Geometry: final body of the model. Coordinates: model frame, mm. Face numbers are marked on the shaded views. Coordinates: 2 decimals unless noted, no trailing zeros. Order: outer loops, then holes, each group sorted by start corner. A loop starts at its lowest first (then second) coordinate and runs counter-clockwise, first axis right, second up. Notation, with made-up numbers: (-6.5, 56) - (23.5, 56) arc R20 ccw to (23.5, 68) - close; hole circle Ø2 at (83.5, 4.5). An arc over 180 degrees is marked (long way). Use a Markdown table: item, result. Add a question column.
```python
from build123d import *

# Parameters (mm, degrees)
SHELL1_T            = -3.81
SKETCH2_R           = 39.624
BOSS_EXTRUDE1_DEPTH = 88.9
SKETCH4_R           = 38.1
CUT_EXTRUDE1_DEPTH  = 88.9
SKETCH5_R           = 34.539650962
CUT_EXTRUDE2_DEPTH  = 575.240692351
SKETCH7_R           = 5.930093594
CUT_EXTRUDE5_DEPTH  = 571.44899759
SKETCH8_R           = 3.175
CUT_EXTRUDE6_DEPTH  = 486.842446429
CIRPATTERN1_COUNT   = 4


with BuildPart() as part:
    # Sketch1 → Revolve1 (revolve)
    with BuildSketch(Plane.XY, mode=Mode.PRIVATE) as revolve1_sk:
        Polygon((0, 0), (-39.624, 0), (0, 635), align=None)
    revolve(revolve1_sk.sketch.rotate(Axis((0, 635, 0), (0, -1, 0)), 180), axis=Axis((0, 635, 0), (0, -1, 0)))


with BuildPart() as body_2:
    # Split1: the piece on the far side of the plane
    add(part.part)
    split(bisect_by=Plane.ZX.offset(482.6), keep=Keep.BOTTOM)

    # Shell1
    shell1_openings = [body_2.faces().sort_by_distance(p)[0] for p in [
        (0, 0, 0),
    ]]
    offset(amount=SHELL1_T, openings=shell1_openings, kind=Kind.INTERSECTION)

    # Sketch2 → Boss-Extrude1 (add)
    with BuildSketch(Plane.XZ):
        Circle(SKETCH2_R)
    extrude(amount=BOSS_EXTRUDE1_DEPTH)

    # Sketch4 → Cut-Extrude1 (cut)
    with BuildSketch(Plane.XZ.offset(88.9)):
        Circle(SKETCH4_R)
    extrude(amount=-CUT_EXTRUDE1_DEPTH, mode=Mode.SUBTRACT)

    # Sketch7 → Cut-Extrude5 (cut, through all)
    with BuildSketch(Plane(origin=(0, 478.79, 0), x_dir=(-1, 0, 0), z_dir=(0, -1, 0))):
        with Locations(Location((0, 0, 0), (0, 0, 90))):
            Circle(SKETCH7_R)
    extrude(amount=-CUT_EXTRUDE5_DEPTH, mode=Mode.SUBTRACT)

    # Sketch8 → Cut-Extrude6 (cut, through all)
    with BuildSketch(Plane(origin=(0, 0, 0), x_dir=(0, 0, -1), z_dir=(1, 0, 0))):
        with Locations(Location((0, -47.625, 0), (0, 0, 270))):
            Circle(SKETCH8_R)
    cut_extrude6 = extrude(amount=CUT_EXTRUDE6_DEPTH, mode=Mode.SUBTRACT)

    # CirPattern1: Cut-Extrude6 ×4 about axis
    cirpattern1_axis = Axis((0, -88.9, 0), (0, 1, 0))
    for i in range(1, CIRPATTERN1_COUNT):
        add(cut_extrude6.rotate(cirpattern1_axis, i * 360 / CIRPATTERN1_COUNT), mode=Mode.SUBTRACT)


with BuildPart() as part_1:
    add(part.part)

    # Split1
    split(bisect_by=Plane.ZX.offset(482.6), keep=Keep.TOP)

    # Sketch5 → Cut-Extrude2 (cut, through all)
    with BuildSketch(Plane(origin=(0, 482.6, 0), x_dir=(1, 0, 0), z_dir=(0, 1, 0))):
        Circle(SKETCH5_R)
    extrude(amount=CUT_EXTRUDE2_DEPTH, mode=Mode.SUBTRACT)


solid = body_2.part
```
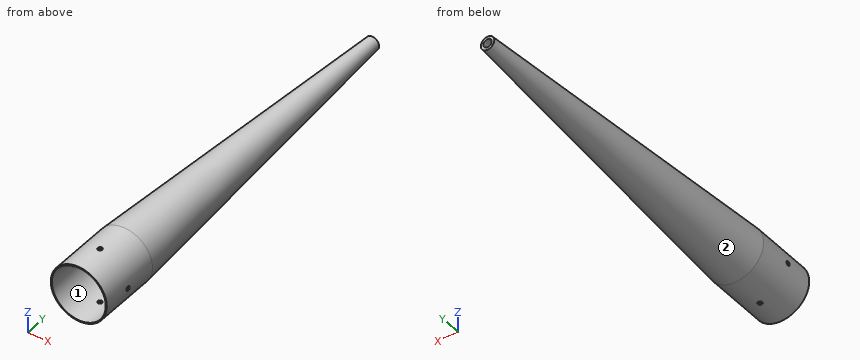
1) Line query: line 1 (Z direction, x = 0, y = -29); line 2 (Z direction, x = -26, y = -45.5); line 3 (X direction, y = 480.8, z = 0). Output: solid intervals per line, ascending. Write a range as from..to.
2) First-contact query: pin 1 (1.5 mm diameter, centred on x = -3.5, y = 153.5, fed in from +Z); pin 2 (6 mm diameter, centred on x = 2, y = 120, fed in from -Z); pin 3 (5 mm diameter, centred on y = 176.5, z = 13.5, fed in from +X). Flat tips, straight axial feed; report the tip coordinate or a pass-through.
3) Section query B-B (y = 287.5). Return the cut outline in (x, z), and give its area (3 significant figures).
4) Draft query along X for the marked faces 1 and 2. Return one class per face: released by +X, released by -X, zero draft, split by the parting line, or undercut.
5) Section query A-A (y = 81). Return the cut outline in (x, z), and give its area (3 significant figures).
From the geometry:
| question | item | result |
|---|---|---|
| 1 | line 1 | z = -39.62..-38.1, 38.1..39.62 |
| 1 | line 2 | z = -29.9..-27.85, 27.85..29.9 |
| 1 | line 3 | x = -9.62..-5.93, 5.93..9.62 |
| 2 | pin 1 | stops at z = 29.93 |
| 2 | pin 2 | stops at z = -32.3 |
| 2 | pin 3 | stops at x = 26.42 |
| 3 | outline | circle Ø43.37 at (0, 0); hole circle Ø35.73 at (0, 0) |
| 3 | area | 474 mm^2 |
| 4 | face 1 | undercut |
| 4 | face 2 | split by the parting line |
| 5 | outline | circle Ø69.14 at (0, 0); hole circle Ø61.5 at (0, 0) |
| 5 | area | 783 mm^2 |
